Design review of the part built by this model. Coordinates are the model's own, in mm. A direction names the side the tool comes from. Coordinates: 2 decimals unless noted, no trailing zeros. Loops run counter-clockwise (first coordinate to the right, second up) from the corner with the lowest first, then second, coordinate; pieces in that order, holes last. Notation, with made-up numbers: (-19, -24) -> (31, -24) arc R16 ccw to (31, -20) -> close; hole circle Ø10 at (2, 36.25). An arc over 180 degrees is marked (long way). Answer in a Markdown table with one row per item.
```python
from build123d import *

# Parameters (mm, degrees)
F0_W     = 80
F0_H     = 80
F1_DEPTH = 580
F2_W     = 80
F2_H     = 50
F3_DEPTH = 20
F4_W     = 50
F4_H     = 60
F5_DEPTH = 20
F6_W     = 80
F6_H     = 50
F7_DEPTH = 20
F8_W     = 50
F8_H     = 60
F9_DEPTH = 20


with BuildPart() as f1:
    # F0 (on Front) → F1 (new body)
    with BuildSketch(Plane.XZ):
        with Locations((4.566346, -9.518241)):
            Rectangle(F0_W, F0_H)
    extrude(amount=-F1_DEPTH)

    # F2 (on face) → F3 (cut)
    with BuildSketch(Plane.XY.offset(30.481759)):
        with Locations((4.566346, 275)):
            Rectangle(F2_W, F2_H)
    extrude(amount=-F3_DEPTH, mode=Mode.SUBTRACT)

    # F4 (on face) → F5 (cut)
    with BuildSketch(Plane.YZ.offset(44.566346)):
        with Locations((275, -19.518241)):
            Rectangle(F4_W, F4_H)
    extrude(amount=-F5_DEPTH, mode=Mode.SUBTRACT)

    # F6 (on face) → F7 (cut)
    with BuildSketch(Plane.XY.offset(30.481759)):
        with Locations((4.566346, 555)):
            Rectangle(F6_W, F6_H)
    extrude(amount=-F7_DEPTH, mode=Mode.SUBTRACT)

    # F8 (on face) → F9 (cut)
    with BuildSketch(Plane.YZ.offset(44.566346)):
        with Locations((555, -19.518241)):
            Rectangle(F8_W, F8_H)
    extrude(amount=-F9_DEPTH, mode=Mode.SUBTRACT)


solid = f1.part
```
(1) Tool access review of faces 4 (the flat face through (22, 250, 18)), 5 (the flat face through (24.566, 275, -19)), 6 (the flat face through (44.566, 413, -10)), 7 (the flat face through (-6, 555, 10.482)): name each direction out of +Z, -Z, +X, -X, +Y, -Y from which nothing blocks a thin tool from reaching the whole face with its end or side.
Evaluation:
| item | result |
|---|---|
| face 4 | +Z, +X |
| face 5 | +Z, -Z, +X |
| face 6 | +Z, -Z, +X, +Y, -Y |
| face 7 | +Z, +X, -X, +Y |
(2) Take a section at B-B on z = -12.5. Give the boundary of the cut face in (x, y).
Evaluation:
| item | result |
|---|---|
| outline | (-35.43, 0) -> (44.57, 0) -> (44.57, 250) -> (24.57, 250) -> (24.57, 300) -> (44.57, 300) -> (44.57, 530) -> (24.57, 530) -> (24.57, 580) -> (-35.43, 580) -> close |
(3) Take a section at A-A on x = -15. Give the boundary of the cut face in (y, z), and give its area (3 significant figures).
Evaluation:
| item | result |
|---|---|
| outline | (0, -49.52) -> (580, -49.52) -> (580, 10.48) -> (530, 10.48) -> (530, 30.48) -> (300, 30.48) -> (300, 10.48) -> (250, 10.48) -> (250, 30.48) -> (0, 30.48) -> close |
| area | 44,400 mm² |
(4) Draft analysis for pull direction Y (two halves, no side actions). For faces 1 (the flat face through (24.566, 555, -19)), 2 (the flat face through (-6, 275, 10.482)), 3 (the flat face through (4, 0, -9)), state which applies: pulls with the +Y half, pulls with the -Y half, needs draft (parallel to the pull), parting line crosses it, or undercut.
Evaluation:
| item | result |
|---|---|
| face 1 | needs draft |
| face 2 | undercut |
| face 3 | pulls with the -Y half |
(5) Take a section at C-C on y = 261. Give the boundary of the cut face in (x, z).
Evaluation:
| item | result |
|---|---|
| outline | (-35.43, -49.52) -> (24.57, -49.52) -> (24.57, 10.48) -> (-35.43, 10.48) -> close |
(6) For pin 1 (15 mm diameter, centred on y = 272, z = -7.5, fed in from +X); pin 2 (1.5 mm diameter, centred on x = -14.5, z = 18.5, fed in from +Y); pin 3 (15 mm diameter, centred on x = -1, y = 282.5, fed in from +Z), all flat-tipped, find the tip position at first contact; note any pin that passes through.
Evaluation:
| item | result |
|---|---|
| pin 1 | stops at x = 24.57 |
| pin 2 | stops at y = 530 |
| pin 3 | stops at z = 10.48 |
(7) To check wall thickness, follow probe 1 along Y at (x, z) = (30.5, 6); probe 2 along X at (y, z) = (286, -9.5); probe 3 along Z at (x, y) = (18.5, 277.5). State the ranges of each line that lie inside material, in increasing order.
Evaluation:
| item | result |
|---|---|
| probe 1 | y = 0 to 250, 300 to 530 |
| probe 2 | x = -35.43 to 24.57 |
| probe 3 | z = -49.52 to 10.48 |
